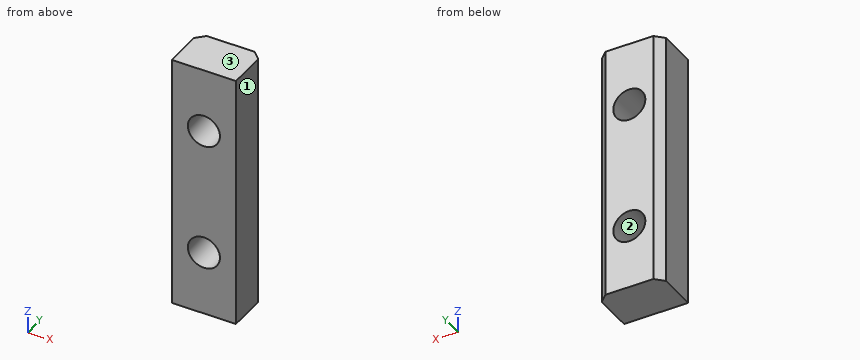
Autodesk Fusion 360 part; units mm, degrees
sketch "Sketch1" plane through (0, 0, 0) normal (0, 1, 0) x (1, 0, 0)
  line L0 (2, -8) -> (-2, -8)
  line L1 (-2, -8) -> (-2, 8)
  line L2 (-2, 8) -> (2, 8)
  line L3 (2, 8) -> (2, -8)
  line L4 (0, 3.9919) -> (0, -4.0081) construction
  circle A0 centre (0, 3.9919) radius 1
  circle A1 centre (0, -4.0081) radius 1
  dimension "d1" = 16
  dimension "d2" = 4
  dimension "d3" = 8
  dimension "d4" = 2
  dimension "d5" = 2
extrude "Extrude1" add sketch "Sketch1" along normal blind 2.9
chamfer "Chamfer1" distance 0.5 angle 45 1 edges at (2, 2.9, 0)
chamfer "Chamfer2" distance 0.5 angle 45 1 edges at (-2, 2.9, 0)
thread "Thread1"
thread "Thread2"
The model under review builds one solid part; all positions refer to its coordinate system, in mm. Face numbers are marked on the shaded views. Give positions to 0.01 mm unless a question says otherwise; leave off trailing zeros. Loops run counter-clockwise (first coordinate to the right, second up) from the corner with the lowest first, then second, coordinate; pieces in that order, holes last. Notation, with made-up numbers: (3.25, 10) - (10.25, 10) arc R35 cw to (10.25, 43) - close; hole circle Ø9 at (88, 89.25). An arc over 180 degrees is marked (long way). Answer as a JSON object with one key per item and string values.
Q1. Add section D-D on y = 0.35. State the section outline as (x, z) points, plus the area to 3 significant figures.
Worked out:
{"outline": "(-2, -8) - (2, -8) - (2, 8) - (-2, 8) - close; hole circle Ø2 at (0, -3.99); hole circle Ø2 at (0, 4.01)", "area": "57.7 mm^2"}
Q2. Mouldability with a two-part tool opening along X and no side actions: class the marked faces 1, 2 and 3 as +X half, -X half, draft (parallel to the pull), parting line (faces both ways), or undercut.
Worked out:
{"face 1": "+X half", "face 2": "undercut", "face 3": "draft"}
Q3. To check wall thickness, follow line 1 along Z through (x, y) = (0, 1.25); line 2 along X through (y, z) = (1.8, 4.5); line 3 along X through (y, z) = (2.8, -4.25). State the ranges of each line that lie inside material, in increasing order.
Worked out:
{"line 1": "z = -8 to -4.99, -2.99 to 3.01, 5.01 to 8", "line 2": "x = -2 to -0.87, 0.87 to 2", "line 3": "x = -1.6 to -0.97, 0.97 to 1.6"}
Q4. Add section B-B on z = 6. State the section outline as (x, y) points, plus the area to 4 significant figures.
Worked out:
{"outline": "(-2, 0) - (2, 0) - (2, 2.4) - (1.5, 2.9) - (-1.5, 2.9) - (-2, 2.4) - close", "area": "11.35 mm^2"}
Q5. Add section C-C on x = 0.6. State the section outline as (y, z) points, plus the area to 3 significant figures.
Worked out:
{"outline": "(0, -8) - (2.9, -8) - (2.9, -4.79) - (0, -4.79) - close; (0, -3.19) - (2.9, -3.19) - (2.9, 3.21) - (0, 3.21) - close; (0, 4.81) - (2.9, 4.81) - (2.9, 8) - (0, 8) - close", "area": "37.1 mm^2"}
Q6. Add section A-A on x = 0. State the section outline as (y, z) points, plus the area to 3 significant figures.
Worked out:
{"outline": "(0, -8) - (2.9, -8) - (2.9, -4.99) - (0, -4.99) - close; (0, -2.99) - (2.9, -2.99) - (2.9, 3.01) - (0, 3.01) - close; (0, 5.01) - (2.9, 5.01) - (2.9, 8) - (0, 8) - close", "area": "34.8 mm^2"}
Q7. Insertion check: pin 1 (2 mm diameter, centred on x = 0.5, z = 5, fed in from -Y); pin 2 (1.2 mm diameter, centred on x = 0, z = 4.01, fed in from +Y). Each pin has a flat end and moves straight along its axis. Give the tip position at first contact, or say it passes through.
Worked out:
{"pin 1": "stops at y = 0", "pin 2": "passes through"}
